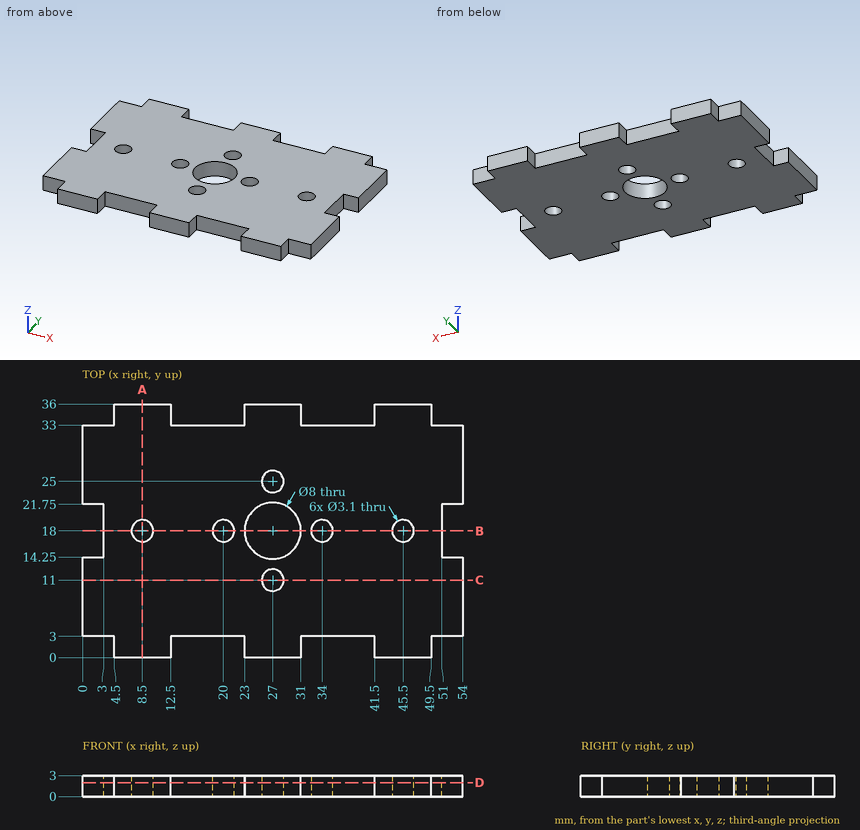
Design review of the part shown in the three views and the two pictorial views. Dimensions are in mm from the part's minimum x, y and z. Round coordinates to 2 decimals unless told otherwise and drop trailing zeros. Order: outer loops, then holes, each group sorted by start corner. A loop starts at its lowest first (then second) coordinate and runs counter-clockwise, first axis right, second up.
Item 1: Add section A-A, the plane x = 8.5. State the section outline as (y, z) points.
Working result:
outline: (0, 0) - (16.45, 0) - (16.45, 3) - (0, 3) - close; (19.55, 0) - (36, 0) - (36, 3) - (19.55, 3) - close
Item 2: Add section B-B, the plane y = 18. State the section outline as (x, z) points.
Working result:
outline: (3, 0) - (6.95, 0) - (6.95, 3) - (3, 3) - close; (10.05, 0) - (18.45, 0) - (18.45, 3) - (10.05, 3) - close; (21.55, 0) - (23, 0) - (23, 3) - (21.55, 3) - close; (31, 0) - (32.45, 0) - (32.45, 3) - (31, 3) - close; (35.55, 0) - (43.95, 0) - (43.95, 3) - (35.55, 3) - close; (47.05, 0) - (51, 0) - (51, 3) - (47.05, 3) - close
Item 3: Add section C-C, the plane y = 11. State the section outline as (x, z) points.
Working result:
outline: (0, 0) - (25.45, 0) - (25.45, 3) - (0, 3) - close; (28.55, 0) - (54, 0) - (54, 3) - (28.55, 3) - close
Item 4: To check wall thickness, follow probe 1 along Y at (x, z) = (27, 1.9); probe 2 along X at (y, z) = (18, 2.3); probe 3 along Y at (x, z) = (20, 0.7). State the ranges of each line that lie inside material, in increasing order.
Working result:
probe 1: y = 0 to 9.45, 12.55 to 14, 22 to 23.45, 26.55 to 36
probe 2: x = 3 to 6.95, 10.05 to 18.45, 21.55 to 23, 31 to 32.45, 35.55 to 43.95, 47.05 to 51
probe 3: y = 3 to 16.45, 19.55 to 33
Item 5: Add section D-D, the plane z = 2. Count the separate pieces of the cut face and the enclosed holes in it, and give its area (3 significant figures).
Working result:
separate pieces: 1
enclosed holes: 7
area: 1,620 mm2
Item 6: For pin 1 (3 mm diameter, centred on x = 45.5, y = 18, fed in from -Z); pin 2 (1.5 mm diameter, centred on x = 18, z = 2, fed in from -Y); pin 3 (0.9 mm diameter, centred on y = 2, z = 1.5, fed in from -X); pin 4 (0.9 mm diameter, centred on y = 16.5, z = 1.5, fed in from -X), all flat-tipped, find the tip position at first contact; note any pin that passes through.
Working result:
pin 1: passes through
pin 2: stops at y = 3
pin 3: stops at x = 4.5
pin 4: stops at x = 3
